Part print with two shaded views. Sizes in mm from the minimum x, y, z corner. A direction names the side the tool comes from. Coordinates: 2 decimals unless noted, no trailing zeros. Order: outer loops, then holes, each group sorted by start corner. A loop starts at its lowest first (then second) coordinate and runs counter-clockwise, first axis right, second up. Notation, with made-up numbers: (38, 7) - (61, 7) arc R26 ccw to (61, 36) - close; hole circle Ø8 at (-26.75, -2). An arc over 180 degrees is marked (long way). Return JSON: item names as keys, results as strings.
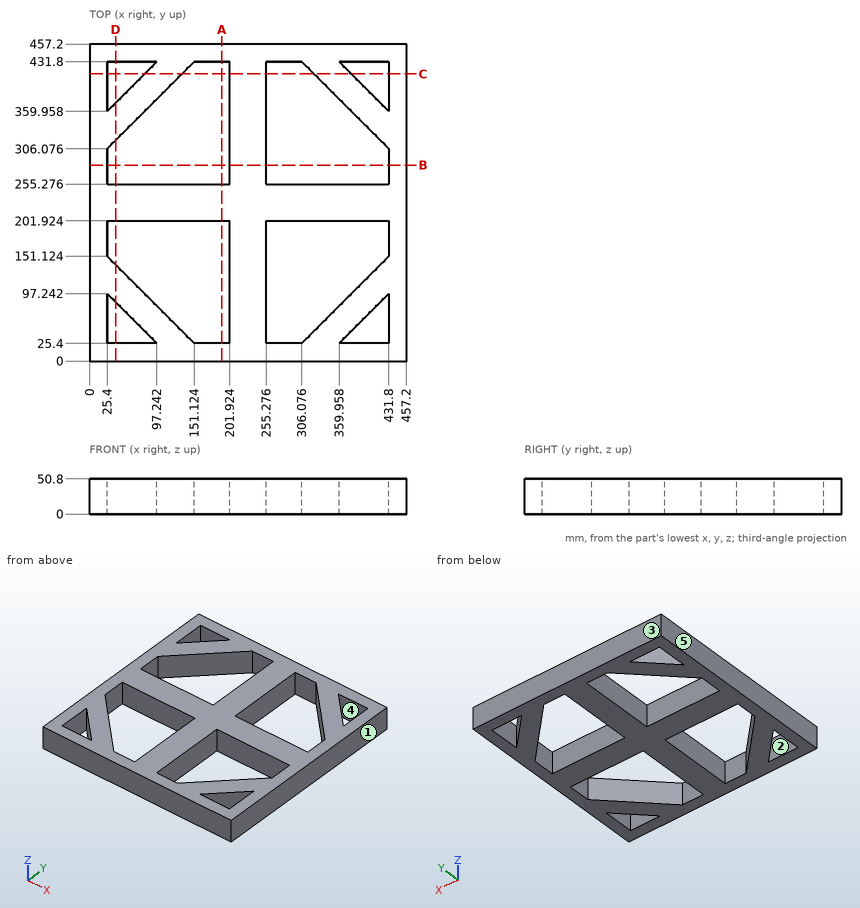
Item 1: Which spindle directions (+Z, -Z, +X, -X, +Y, -Y) get a long thin tool onto all of the face, cutting with end or side? Do the marked faces 1 and 2. Say none if no direction does.
Findings below:
{"face 1": "+Z, -Z, +X, +Y, -Y", "face 2": "+Z, -Z"}
Item 2: Band-saw the part on C-C, the plane y = 414. List the corners of the cut face in (x, z).
Findings below:
{"outline": "(0, 0) - (25.4, 0) - (25.4, 50.8) - (0, 50.8) - close; (79.44, 0) - (133.32, 0) - (133.32, 50.8) - (79.44, 50.8) - close; (201.92, 0) - (255.28, 0) - (255.28, 50.8) - (201.92, 50.8) - close; (323.88, 0) - (377.76, 0) - (377.76, 50.8) - (323.88, 50.8) - close; (431.8, 0) - (457.2, 0) - (457.2, 50.8) - (431.8, 50.8) - close"}
Item 3: Mould opens along Y. For the marked faces 3, 4 and 5 say: released by +Y, released by -Y, zero draft, split by the parting line, or undercut.
Findings below:
{"face 3": "released by +Y", "face 4": "undercut", "face 5": "zero draft"}
Item 4: Wall check: L1, parallel to Y at x = 285, z = 21; L2, parallel to Y at x = 423, z = 20 (1 decimal). Give the ranges that are in metal, low to high. Write a range as [from, to].
Findings below:
{"L1": "y = [0, 25.4], [201.92, 255.28], [431.8, 457.2]", "L2": "y = [0, 25.4], [88.4, 142.3], [201.9, 255.3], [314.9, 368.8], [431.8, 457.2]"}
Item 5: Band-saw the part on D-D, the plane x = 37.5. List the corners of the cut face in (y, z).
Findings below:
{"outline": "(0, 0) - (25.4, 0) - (25.4, 50.8) - (0, 50.8) - close; (85.14, 0) - (139.02, 0) - (139.02, 50.8) - (85.14, 50.8) - close; (201.92, 0) - (255.28, 0) - (255.28, 50.8) - (201.92, 50.8) - close; (318.18, 0) - (372.06, 0) - (372.06, 50.8) - (318.18, 50.8) - close; (431.8, 0) - (457.2, 0) - (457.2, 50.8) - (431.8, 50.8) - close"}
Item 6: Band-saw the part on A-A, the plane x = 191. List the corners of the cut face in (y, z), then the cut area to 3 significant figures.
Findings below:
{"outline": "(0, 0) - (25.4, 0) - (25.4, 50.8) - (0, 50.8) - close; (201.92, 0) - (255.28, 0) - (255.28, 50.8) - (201.92, 50.8) - close; (431.8, 0) - (457.2, 0) - (457.2, 50.8) - (431.8, 50.8) - close", "area": "5,290 mm²"}
